from build123d import *

# Parameters (mm, degrees)
F1_DEPTH = 6
F2_R     = 6.5
F3_DEPTH = 6
F5_DEPTH = 6


with BuildPart() as f1:
    # F0 (on Front) → F1 (new body)
    with BuildSketch(Plane.XZ):
        with BuildLine():
            Line((12.5, -32), (12.5, 32))
            Line((12.5, 32), (-12.5, 32))
            Line((-12.5, 32), (-12.5, -32))
            Line((-12.5, -32), (-6.5, -32))
            Line((-6.5, -32), (-6.5, -12))
            ThreePointArc((-6.5, -12), (0, -5.5), (6.5, -12))
            Line((6.5, -12), (6.5, -32))
            Line((6.5, -32), (12.5, -32))
        make_face()
    extrude(amount=F1_DEPTH)

    # F2 (on face) → F3 (join)
    with BuildSketch(Plane.XY.offset(32)):
        with BuildLine():
            Line((-12.5, -6), (12.5, -6))
            Line((12.5, -6), (12.5, 12))
            ThreePointArc((12.5, 12), (0, -0.5), (-12.5, 12))
            Line((-12.5, 12), (-12.5, -6))
        make_face()
        with BuildLine():
            ThreePointArc((-12.5, 12), (0, -0.5), (12.5, 12))
            ThreePointArc((12.5, 12), (0, 24.5), (-12.5, 12))
        make_face()
        with Locations((0, 12)):
            Circle(F2_R, mode=Mode.SUBTRACT)
    extrude(amount=-F3_DEPTH)

    # F4 (on face) → F5 (join)
    with BuildSketch(Plane(origin=(-12.5, 0, 0), x_dir=(0, -1, 0), z_dir=(-1, 0, 0))):
        with BuildLine():
            ThreePointArc((18, 7), (30.5, 19.5), (18, 32))
            Line((18, 32), (18, 26))
            ThreePointArc((18, 26), (22.596194, 24.096194), (24.5, 19.5))
            ThreePointArc((24.5, 19.5), (22.596194, 14.903806), (18, 13))
            Line((18, 13), (18, 7))
        make_face()
        with BuildLine():
            Line((18, 32), (6, 32))
            Line((6, 32), (6, 7))
            Line((6, 7), (18, 7))
            Line((18, 7), (18, 13))
            ThreePointArc((18, 13), (11.5, 19.5), (18, 26))
            Line((18, 26), (18, 32))
        make_face()
    extrude(amount=-F5_DEPTH)


solid = f1.part
Verification items for the finished model (mm, model axes). A direction names the side the tool comes from. Round coordinates to 2 decimals unless told otherwise and drop trailing zeros. Write each loop counter-clockwise with the first axis right and the second up, starting at its lowest first coordinate (ties: lowest second). Pieces come first, ordered by that corner, then holes.
(1) Section check A-A (z = -23). Enter the section's corners in (x, y).
Returned:
outline: (-12.5, -6) - (-6.5, -6) - (-6.5, 0) - (-12.5, 0) - close; (6.5, -6) - (12.5, -6) - (12.5, 0) - (6.5, 0) - close
(2) Material ranges on line 1 (Y direction, x = 0, z = 29.55); line 2 (Y direction, x = 10.75, z = -5); line 3 (X direction, y = 8, z = 28.5), recorded low to high.
Returned:
line 1: y = -6 to 5.5, 18.5 to 24.5
line 2: y = -6 to 0
line 3: x = -12.5 to -5.12, 5.12 to 12.5
(3) Mould release check, pull along X, two halves, no side actions. Record for faces 1 (the flat face through (9, -3, -32)), 2 (the cylindrical face through (-0.1, -3, -5.5)), 3 (the flat face through (12.5, -1, 7)), 4 (the flat face through (-12.5, -8, 12)): pulls with the +X half, pulls with the -X half, needs draft (parallel to the pull), parting line crosses it, or undercut.
Returned:
face 1: needs draft
face 2: undercut
face 3: pulls with the +X half
face 4: pulls with the -X half
(4) Access from +Z, -Z, +X, -X, +Y, -Y to the whole of each face (thin tool, end or side, straight path). Record for faces 5 (the flat face through (0, 4, 26)), 6 (the cylindrical face through (-9.542, -30.497, 19.225)), 7 (the flat face through (-6.5, -3, -22)), 8 (the flat face through (-10, -12, 7)), 9 (the flat face through (-6.5, -13, 14)).
Returned:
face 5: -Z, +X, -X, +Y
face 6: +X, -X, -Y
face 7: -Z, +Y, -Y
face 8: -Z, +X, -X, -Y
face 9: +Z, -Z, +X, -Y
(5) Section check B-B (x = 0). Enter the section's corners in (y, z).
Returned:
outline: (-6, -5.5) - (0, -5.5) - (0, 26) - (5.5, 26) - (5.5, 32) - (-6, 32) - close; (18.5, 26) - (24.5, 26) - (24.5, 32) - (18.5, 32) - close
(6) Depth check by flat-ended pin: pin 1 Ø5 at (x, z) = (4.5, -10) entering from -Y; pin 2 Ø7.5 at (x, y) = (4.5, 15) entering from -Z; pin 3 Ø10 at (x, y) = (0.5, -22.5) entering from -Z; pin 4 Ø3 at (x, z) = (-3, 17) entering from +Y. Enter the tip coordinate at first touch or a pass-through.
Returned:
pin 1: stops at y = -6
pin 2: stops at z = 26
pin 3: passes through
pin 4: stops at y = 0
(7) Section check D-D (z = 28.5). Enter the section's corners in (x, y), plus the area to 3 significant figures.
Returned:
outline: (-12.5, -26.67) - (-6.5, -26.67) - (-6.5, -6) - (12.5, -6) - (12.5, 12) arc R12.5 ccw to (-12.5, 12) - close; hole circle Ø13 at (0, 12)
area: 687 mm2
(8) Section check C-C (y = 13). Enter the section's corners in (x, z).
Returned:
outline: (-12.46, 26) - (-6.42, 26) - (-6.42, 32) - (-12.46, 32) - close; (6.42, 26) - (12.46, 26) - (12.46, 32) - (6.42, 32) - close
